Check sheet for the modelled part. Datum: model origin and axes. Units: mm. A direction names the side the tool comes from. Give positions to 0.01 mm unless a question says otherwise; leave off trailing zeros. Order: outer loops, then holes, each group sorted by start corner. A loop starts at its lowest first (then second) coordinate and runs counter-clockwise, first axis right, second up. Notation, with made-up numbers: (-25, 4.5) -> (-16, 4.5) arc R19 ccw to (-16, 34.5) -> close; hole circle Ø10 at (86, -35.5). An arc over 180 degrees is marked (long way). One line per question, with ' | ' between items. Start each with the question number.
from build123d import *

# Parameters (mm, degrees)
F0_W     = 40
F0_H     = 40
F1_DEPTH = 45
F3_R     = 12.5
F4_DEPTH = 30
F2_R     = 12.5
F5_DEPTH = 30
F6_R     = 2.5
F7_DEPTH = 45.001


with BuildPart() as f1:
    # F0 (on Top) → F1 (new body)
    with BuildSketch(Plane.XY):
        with Locations((1.391534, -6.178061)):
            Rectangle(F0_W, F0_H)
    extrude(amount=F1_DEPTH)

    # F3 (on face) → F4 (cut)
    with BuildSketch(Plane.XZ.offset(26.178061)):
        with Locations((1.391534, 25.5)):
            Circle(F3_R)
    extrude(amount=-F4_DEPTH, mode=Mode.SUBTRACT)

    # F2 (on face) → F5 (cut)
    with BuildSketch(Plane(origin=(-18.608466, 0, 0), x_dir=(0, -1, 0), z_dir=(-1, 0, 0))):
        with Locations((6.178061, 25.5)):
            Circle(F2_R)
    extrude(amount=-F5_DEPTH, mode=Mode.SUBTRACT)

    # F6 (on face) → F7 (cut, through all)
    with BuildSketch(Plane.XY.offset(45)):
        with Locations((1.391534, -6.178061)):
            Circle(F6_R)
    extrude(amount=-F7_DEPTH, mode=Mode.SUBTRACT)


solid = f1.part
1. Cross-section at A-A on z = 25.5. Record the boundary of the cut face in (x, y), and give its area (3 significant figures).
2. Mould release check, pull along X, two halves, no side actions. Record for faces 4 (the face through (2.545, -8.396, 41.487)), 5 (the face through (11.392, -6, 35)), 6 (the face through (-3, -6, 45)): +X half, -X half, draft (parallel to the pull), parting line (faces both ways), or undercut.
3. Scan lines: probe 1 along Z at (x, y) = (-4.5, -6.5); probe 2 along Y at (x, z) = (-10.5, 18); probe 3 along Y at (x, z) = (-4.5, 25.5). Record each from-to range of solid material in increasing order.
4. Go/stop test with flat-tipped pins: pin 1 (10 mm diameter, centred on x = 10, y = -0.5, fed in from -Z); pin 2 (2.5 mm diameter, centred on x = 0, z = 14.5, fed in from -Y); pin 3 (1 mm diameter, centred on y = -4, z = 19.5, fed in from -X); pin 4 (1.5 mm diameter, centred on y = -1, z = 34.5, fed in from -X). Record where each tip stops, or that it passes through.
5. Tool access check on faces 1 (the face through (8, -6, 13)), 2 (the face through (1, 3.822, 35)), 3 (the face through (2.545, -8.396, 6.655)). Record the directions out of +Z, -Z, +X, -X, +Y, -Y that give a thin tool (end or side, any length) a straight path to the whole face; none if there is none.
6. Cross-section at C-C on y = -5. Record the boundary of the cut face in (x, z).
7. Cross-section at B-B on y = -20. Record the boundary of the cut face in (x, z), and give its area (3 significant figures).
8. Cross-section at D-D on x = 4.5. Record the boundary of the cut face in (y, z), and give its area (3 significant figures).
Response values:
1) outline: (-18.61, -26.18) -> (-11.11, -26.18) -> (-11.11, -18.68) -> (-18.61, -18.68) -> close; (-18.61, 6.32) -> (11.39, 6.32) -> (11.39, 3.82) -> (13.89, 3.82) -> (13.89, -26.18) -> (21.39, -26.18) -> (21.39, 13.82) -> (-18.61, 13.82) -> close | area: 606 mm²
2) face 4: undercut | face 5: -X half | face 6: draft
3) probe 1: z = 0 to 13, 38 to 45 | probe 2: y = -26.18 to -16.18, 3.82 to 13.82 | probe 3: y = 6.32 to 13.82
4) pin 1: stops at z = 0 | pin 2: stops at y = 3.82 | pin 3: stops at x = 12.07 | pin 4: stops at x = 11.39
5) face 1: -X | face 2: -Y | face 3: +Z, -Z
6) outline: (-18.61, 0) -> (-0.81, 0) -> (-0.81, 13.06) -> (-18.61, 13.06) -> close; (-18.61, 37.94) -> (-0.81, 37.94) -> (-0.81, 45) -> (-18.61, 45) -> close; (3.6, 0) -> (21.39, 0) -> (21.39, 45) -> (3.6, 45) -> (3.6, 37.94) -> (11.39, 37.94) -> (11.39, 33) arc R12.5 cw to (11.39, 18) -> (11.39, 13.06) -> (3.6, 13.06) -> close
7) outline: (-18.61, 0) -> (21.39, 0) -> (21.39, 45) -> (-18.61, 45) -> close; hole circle Ø25 at (1.39, 25.5) | area: 1,310 mm²
8) outline: (-26.18, 0) -> (13.82, 0) -> (13.82, 45) -> (-26.18, 45) -> (-26.18, 37.61) -> (-9.29, 37.61) arc R12.5 cw to (-3.07, 37.61) -> (3.82, 37.61) -> (3.82, 33) arc R12.5 cw to (3.82, 18) -> (3.82, 13.39) -> (-3.07, 13.39) arc R12.5 cw to (-9.29, 13.39) -> (-26.18, 13.39) -> close | area: 1,040 mm²
